Autodesk Inventor part; units mm, degrees
ref_plane "YZ Plane" through (0, 0, 0) normal (1, 0, 0) x (0, 1, 0)
ref_plane "XZ Plane" through (0, 0, 0) normal (0, 1, 0) x (-1, 0, 0)
ref_plane "XY Plane" through (0, 0, 0) normal (0, 0, 1) x (1, 0, 0)
sketch "Sketch1" plane through (0, 0, 0) normal (0, 0, 1) x (1, 0, 0)
  line L0 (-165.5, 118.75) -> (165.5, 118.75)
  line L1 (165.5, 118.75) -> (165.5, -118.75)
  line L2 (165.5, -118.75) -> (-165.5, -118.75)
  line L3 (-165.5, -118.75) -> (-165.5, 118.75)
  point P0 (0, 0)
  point P1 (-165.5, 0)
  point P2 (0, 118.75)
  dimension "d0" = 331
  dimension "d2" = 237.5
extrude "Extrusion1" add sketch "Sketch1" along normal blind 12.5
sketch "Sketch2" plane through (0, 0, 0) normal (0, 0, -1) x (-1, 0, 0)
  circle A0 centre (-150.5, 103.75) radius 1.55
  line L0 (-145.8379, -108.9576) -> (-147.4259, -106.1413)
  circle A1 centre (150.5, -108.75) radius 1.55
  circle A2 centre (150.5, 103.75) radius 1.55
  line L1 (150.5, -108.75) -> (-150.5, -108.75)
  line L2 (-150.5, -108.75) -> (-150.5, 103.75)
  line L3 (-150.5, 103.75) -> (150.5, 103.75)
  line L4 (150.5, 103.75) -> (150.5, -108.75)
  circle A3 centre (-150.5, -108.75) radius 1.55
  point P0 (0, 0)
extrude "Extrusion2" cut sketch "Sketch2" against normal through all contours L3 L2 A0 | A0 L2 L3 | L3 L4 A2 | A2 L4 L3 | A3 L1 L2 | L2 L1 A3 | L4 L1 A1 | A1 L1 L4
sketch "Sketch3" plane through (0, 0, 0) normal (0, 0, -1) x (-1, 0, 0)
  circle A0 centre (150.5, -108.75) radius 1.55
  circle A1 centre (-150.5, 103.75) radius 1.55
  circle A2 centre (-150.5, -108.75) radius 1.55
  circle A3 centre (150.5, 103.75) radius 1.55
  circle A4 centre (-150.5, 103.75) radius 3.25
  circle A5 centre (-150.5, -108.75) radius 3.25
  circle A6 centre (150.5, -108.75) radius 3.25
  circle A7 centre (150.5, 103.75) radius 3.25
  circle A8 centre (-150.5, -108.75) radius 1.55
  point P0 (0, 0)
  dimension "d7" = 6.5
hole "Hole1" at (150.5, 103.75, 0) at (150.5, -108.75, 0) at (-150.5, -108.75, 0) at (-150.5, 103.75, 0) direction (0, 0, 1) diameter 3.4 end through all counterbore diameter 6.5 counterbore depth 3
sketch "Sketch4" plane through (0, 0, 0) normal (0, 0, -1) x (-1, 0, 0)
  circle A0 centre (-2, -73.75) radius 1.621
  circle A1 centre (48, 76.25) radius 1.621
  circle A2 centre (-2, 76.25) radius 1.621
  circle A3 centre (48, -73.75) radius 1.621
  line L0 (-34.5, 108.75) -> (-34.5, -106.25)
  line L1 (-34.5, -106.25) -> (80.5, -106.25)
  line L2 (80.5, -106.25) -> (80.5, 108.75)
  line L3 (80.5, 108.75) -> (-34.5, 108.75)
  point P0 (0, 0)
hole "Hole2" at (-48, -73.75, 0) at (2, -73.75, 0) at (-48, 76.25, 0) at (2, 76.25, 0) direction (0, 0, 1) diameter 4.5 end through all counterbore diameter 8 counterbore depth 4
sketch "Sketch5" plane through (0, 0, 0) normal (0, 0, -1) x (-1, 0, 0)
  circle A0 centre (-143.139, 21.4425) radius 1.7
  circle A1 centre (-52.461, 65.2575) radius 1.7
  circle A2 centre (-143.139, 65.2575) radius 1.7
  circle A3 centre (-52.461, 21.4425) radius 1.7
  line L0 (-47, 17.95) -> (-148.6, 17.95)
  line L1 (-47, 68.75) -> (-47, 17.95)
  line L2 (-148.6, 68.75) -> (-47, 68.75)
  line L3 (-148.6, 17.95) -> (-148.6, 68.75)
  point P0 (0, 0)
hole "Hole3" at (143.139, 65.2575, 0) at (143.139, 21.4425, 0) at (52.461, 65.2575, 0) at (52.461, 21.4425, 0) direction (0, 0, 1) diameter 3.4 end through all counterbore diameter 6.5 counterbore depth 3
properties part number "bottom"
CAD build for the part. Positions are in the model's coordinates, mm. A direction names the side the tool comes from. Coordinates: 2 decimals unless noted, no trailing zeros. Use CSV: the item, a comma, the result in double quotes. Start each with the question number.
Item 1: Tool access for faces 1 (the flat face through (-165.5, -2, 6)), 2 (the cylindrical face through (148.303, 101.355, 1.521)): list every direction of +Z, -Z, +X, -X, +Y, -Y with a clear straight run to the whole face (end or side of a thin tool).
Item 2: Wall check: probe 1 along X at (y, z) = (76.25, 1.95); probe 2 along Y at (x, z) = (-150.5, 1.85); probe 3 along X at (y, z) = (22.5, 11.5). Give the ranges that are in metal, low to high.
Item 3: Drop flat-ended pins along their axis: P1, Ø3, axis at x = -150.5, y = 103.75, coming from the +Z side; P2, Ø2, axis at x = -150.5, y = -107.5, coming from the -Z side. Give the stop position or say it passes through.
Item 4: Two-plate mould, pull along X, no slides. Class faces 3 (the cylindrical face through (51.48, 24.54, 1.52)), 4 (the flat face through (-2, 2, 12.5)), 5 (the flat face through (165.5, 2, 6)): +X half, -X half, draft (parallel to the pull), parting line (faces both ways), or undercut.
Response values:
1,face 1,"+Z, -Z, -X, +Y, -Y"
1,face 2,"-Z"
2,probe 1,"x = -165.5 to -52, -44 to -2, 6 to 165.5"
2,probe 2,"y = -118.75 to -112, -105.5 to 100.5, 107 to 118.75"
2,probe 3,"x = -165.5 to 51.13, 53.79 to 141.81, 144.47 to 165.5"
3,P1,"passes through"
3,P2,"stops at z = 3"
4,face 3,"undercut"
4,face 4,"draft"
4,face 5,"+X half"
